CAD build for the part. Positions are in the model's coordinates, mm. A direction names the side the tool comes from. Give positions to 0.01 mm unless a question says otherwise; leave off trailing zeros. Order: outer loops, then holes, each group sorted by start corner. A loop starts at its lowest first (then second) coordinate and runs counter-clockwise, first axis right, second up.
Item 1: Wall check: L1, parallel to X at y = -9.25, z = 20; L2, parallel to Z at x = -2, y = -11.25; L3, parallel to X at y = -3.5, z = -14.5. Give the ranges that are in metal, low to high.
Item 2: Which spindle directions (+Z, -Z, +X, -X, +Y, -Y) get a long thin tool onto all of the face, cutting with end or side? Do faces 5 (the flat face through (-25.4, -13, 19)), 6 (the flat face through (41, -13, -12.7)), 7 (the flat face through (-38, -13, 25.4)). Say none if no direction does.
Item 3: Band-saw the part on A-A on y = -22.5. Give the cut face in (x, z), plus the area to 3 significant figures.
Item 4: Two-plate mould, pull along Z, no slides. Class faces 1 (the cylindrical face through (38.28, -6.13, -0.39)), 2 (the flat face through (25.4, -12, 2)), 3 (the flat face through (-10, -13, -25.4)), 4 (the flat face through (31.75, -13, -19)): released by +Z, released by -Z, zero draft, split by the parting line, or undercut.
Item 5: Flat gauge pin, fed straight in: P1, Ø8, axis at y = -19, z = -19.5, coming from the +X side. Where does the tip first touch, or does it go through?
Item 6: Band-saw the part on C-C on x = 17.5. Give the cut face in (y, z).
Item 7: Band-saw the part on D-D on x = 35. Give the cut face in (y, z), plus the area to 3 significant figures.
Item 8: Band-saw the part on B-B on z = 6. Give the cut face in (x, y).
```python
from build123d import *

# Parameters (mm, degrees)
F0_W     = 101.6
F0_H     = 50.8
F1_DEPTH = 25.4
F2_W     = 50.8
F2_H     = 12.7
F3_DEPTH = 25.401
F4_W     = 25.4
F4_H     = 12.7
F5_DEPTH = 19.05
F6_R     = 6.35
F7_DEPTH = 25.4


with BuildPart() as f1:
    # F0 (on Front) → F1 (new body)
    with BuildSketch(Plane.XZ):
        Rectangle(F0_W, F0_H)
    extrude(amount=F1_DEPTH)

    # F2 (on face) → F3 (cut, through all)
    with BuildSketch(Plane.XZ.offset(25.4)):
        with Locations((0, 19.05)):
            Rectangle(F2_W, F2_H)
    extrude(amount=-F3_DEPTH, mode=Mode.SUBTRACT)

    # F4 (on face) → F5 (cut)
    with BuildSketch(Plane.YZ.offset(50.8)):
        with Locations((-12.7, -19.05)):
            Rectangle(F4_W, F4_H)
    extrude(amount=-F5_DEPTH, mode=Mode.SUBTRACT)

    # F6 (on face) → F7 (cut)
    with BuildSketch(Plane.YZ.offset(50.8)):
        with Locations((-11.998156, 2.038684)):
            Circle(F6_R)
    extrude(amount=-F7_DEPTH, mode=Mode.SUBTRACT)


solid = f1.part
```
The answers:
1. L1: x = -50.8 to -25.4, 25.4 to 50.8
1. L2: z = -25.4 to 12.7
1. L3: x = -50.8 to 31.75
2. face 5: +Z, +Y, -Y
2. face 6: -Z, +X, +Y, -Y
2. face 7: +Z, +X, -X, +Y, -Y
3. outline: (-50.8, -25.4) - (31.75, -25.4) - (31.75, -12.7) - (50.8, -12.7) - (50.8, 25.4) - (25.4, 25.4) - (25.4, 12.7) - (-25.4, 12.7) - (-25.4, 25.4) - (-50.8, 25.4) - close
3. area: 4,270 mm2
4. face 1: undercut
4. face 2: undercut
4. face 3: released by -Z
4. face 4: zero draft
5. P1: stops at x = 31.75
6. outline: (-25.4, -25.4) - (0, -25.4) - (0, 12.7) - (-25.4, 12.7) - close
7. outline: (-25.4, -12.7) - (0, -12.7) - (0, 25.4) - (-25.4, 25.4) - close; hole circle Ø12.7 at (-12, 2.04)
7. area: 841 mm2
8. outline: (-50.8, -25.4) - (50.8, -25.4) - (50.8, -16.96) - (25.4, -16.96) - (25.4, -7.04) - (50.8, -7.04) - (50.8, 0) - (-50.8, 0) - close
